from build123d import *

# Parameters (mm, degrees)
SKETCH1_R                = 4.05
BOSS_EXTRUDE1_DEPTH      = 8.1
BOSS_EXTRUDE2_DEPTH      = 1
FILLET1_R                = 10
SKETCH3_R                = 2
BOSS_EXTRUDE3_DEPTH      = 1.2
SKETCH4_R                = 0.4
BOSS_EXTRUDE4_DEPTH      = 3
BOSS_EXTRUDE5_START      = -0.5
SKETCH5_R                = 1.15
BOSS_EXTRUDE5_DEPTH      = 1.4
BOSS_EXTRUDE6_REACH      = 19.008
BOSS_EXTRUDE6_END_RADIUS = 4.05
SKETCH6_W                = 6
SKETCH6_H                = 4


with BuildPart() as part:
    # Sketch1 → Boss-Extrude1 (new body)
    with BuildSketch(Plane(origin=(0, 0, 0), x_dir=(1, 0, 0), z_dir=(0, 1, 0))):
        with Locations(Location((0, 0, 0), (0, 0, 270))):
            Circle(SKETCH1_R)
    extrude(amount=BOSS_EXTRUDE1_DEPTH)

    # Sketch2 → Boss-Extrude2 (add)
    with BuildSketch(Plane(origin=(0, 8.1, 0), x_dir=(1, 0, 0), z_dir=(0, 1, 0))):
        with BuildLine():
            ThreePointArc((-3.833548742, 1.30629401), (-2.205788092, -3.3966158), (2.752603705, -2.9708034))
            ThreePointArc((2.752603705, -2.9708034), (4.235286368, -2.750427127), (3.833548742, -1.30629401))
            ThreePointArc((3.833548742, -1.30629401), (2.205788092, 3.3966158), (-2.752603705, 2.9708034))
            ThreePointArc((-2.752603705, 2.9708034), (-4.235286368, 2.750427127), (-3.833548742, 1.30629401))
        make_face()
    extrude(amount=BOSS_EXTRUDE2_DEPTH)

    # Fillet1
    # the kernel refuses this fillet: 10 mm, written as the material it adds along each edge
    with BuildSketch(Plane(origin=(-2.752603705, 8.1, -2.9708034), x_dir=(0.8459561601363162, 0, -0.5332524497153475), z_dir=(0, 1, 0)), Plane(origin=(2.752603705, 8.1, 2.9708034), x_dir=(-0.8459561601363164, 0, 0.5332524497153472), z_dir=(0, 1, 0))) as fillet1_piece_1:
        with BuildLine():
            CenterArc((3.326797297, 9.829634829), FILLET1_R, 247.104601823, 12.304164649)
            ThreePointArc((-0.563702324, 0.617468271), (-0.214223286, 0.370473326), (0, 0))
            ThreePointArc((0, 0), (0.74439387, 0.068997894), (1.488787741, 0))
        make_face()
    extrude(amount=1)
    with BuildSketch(Plane(origin=(-3.833548742, 8.1, -1.30629401), x_dir=(-0.14306898445110627, 0, 0.9897127187664757), z_dir=(0, 1, 0)), Plane(origin=(3.833548742, 8.1, 1.30629401), x_dir=(0.14306898445110644, 0, -0.9897127187664757), z_dir=(0, 1, 0))) as fillet1_piece_2:
        with BuildLine():
            CenterArc((3.326797297, -9.829634829), FILLET1_R, 100.591233529, 12.304164649)
            ThreePointArc((-0.563702324, -0.617468271), (-0.214223286, -0.370473326), (0, 0))
            ThreePointArc((0, 0), (0.74439387, -0.068997894), (1.488787741, 0))
        make_face()
    extrude(amount=1)

    # Sketch3 → Boss-Extrude3 (add)
    with BuildSketch(Plane(origin=(0, 9.1, 0), x_dir=(1, 0, 0), z_dir=(0, 1, 0))):
        with Locations(Location((0, 0, 0), (0, 0, 270))):
            Circle(SKETCH3_R)
    extrude(amount=BOSS_EXTRUDE3_DEPTH)

    # Sketch4 → Boss-Extrude4 (add)
    with BuildSketch(Plane(origin=(0, 10.3, 0), x_dir=(1, 0, 0), z_dir=(0, 1, 0))):
        with Locations(Location((0, 0, 0), (0, 0, 270))):
            Circle(SKETCH4_R)
    extrude(amount=BOSS_EXTRUDE4_DEPTH)

    # Sketch5 → Boss-Extrude5 (add)
    with BuildSketch(Plane(origin=(0, 13.3, 0), x_dir=(1, 0, 0), z_dir=(0, 1, 0)).offset(BOSS_EXTRUDE5_START)):
        with Locations(Location((0, 0, 0), (0, 0, 270))):
            Circle(SKETCH5_R)
    extrude(amount=-BOSS_EXTRUDE5_DEPTH)

    # Boss-Extrude6: up to this cylinder (the profile starts outside it)
    boss_extrude6_end = Plane(origin=(0, 3.8, 0), z_dir=(0, -1, 0)) * Cylinder(BOSS_EXTRUDE6_END_RADIUS, 47.116, mode=Mode.PRIVATE)
    # Sketch6 → Boss-Extrude6 (add, up to the surface)
    with BuildSketch(Plane(origin=(5.4, 0, 0), x_dir=(0, 0, -1), z_dir=(1, 0, 0)), mode=Mode.PRIVATE) as boss_extrude6_sk1:
        with Locations((0, 3.8)):
            Rectangle(SKETCH6_W, SKETCH6_H)
    boss_extrude6_tool1 = extrude(boss_extrude6_sk1.sketch, amount=-BOSS_EXTRUDE6_REACH, mode=Mode.PRIVATE) - boss_extrude6_end
    add(boss_extrude6_tool1.solids().sort_by_distance((5.4, 3.8, 0))[0])


solid = part.part
Can you work these out from the model? Positions are in its coordinate system, mm. A direction names the side the tool comes from. Round coordinates to 2 decimals unless told otherwise and drop trailing zeros. Loops run counter-clockwise (first coordinate to the right, second up) from the corner with the lowest first, then second, coordinate; pieces in that order, holes last. Notation, with made-up numbers: (39.5, 23) - (62.5, 23) arc R28 cw to (62.5, 43) - close; hole circle Ø5 at (26, -40). An arc over 180 degrees is marked (long way). Use CSV: the item, a comma, the result in double quotes. Start each with the question number.
1) For pin 1 Ø3 at (x, z) = (4, -1) entering from +Y; pin 2 Ø5 at (x, y) = (3.5, 5) entering from +Z; pin 3 Ø1.5 at (y, z) = (9.5, -0.5) entering from -X, each with a flat end and sliding along its axis, tell me the tip position at first contact or that it passes through.
2) If we section it at A-A on z = 1.5: Write out the boundary of the cut face in (x, y).
3) If we section it at D-D on y = 11.25: Write out the boundary of the cut face in (x, z).
4) Please list where these lines run through material, in increasing order: probe 1 along Y at (x, z) = (1.25, 2.25); probe 2 along Z at (x, y) = (5.25, 2.75); probe 3 along X at (y, z) = (2.75, 1.5). Write a range as [from, to].
5) If we section it at C-C on x = 2.25: Write out the boundary of the cut face in (y, z).
6) For faces 5 (the cylindrical face through (0.345, 12.11, 1.097)), 6 (the cylindrical face through (4.146, 8.593, 0.886)), 7 (the flat face through (-0.5, 11.4, 0.24)), which set-ups out of +Z, -Z, +X, -X, +Y, -Y let a thin tool reach every point of the face, with its end or its side?
7) We'd pull the mould along Y, two halves only. Please class faces 1 (the flat face through (-0.4, 10.3, 0.4)), 2 (the flat face through (-1, 9.1, 2)), 3 (the flat face through (4, 8.1, 2)), 4 (the flat face through (4, 4, -3)): released by +Y, released by -Y, zero draft, split by the parting line, or undercut.
8) If we section it at B-B on x = -1: Write out the boundary of the cut face in (y, z), plus the area to 3 significant figures.
Geometry results:
1,pin 1,"stops at y = 9.1"
1,pin 2,"stops at z = 3.92"
1,pin 3,"stops at x = -4.19"
2,outline,"(-3.76, 0) - (3.76, 0) - (3.76, 1.8) - (5.4, 1.8) - (5.4, 5.8) - (3.76, 5.8) - (3.76, 8.1) - (4.26, 8.1) - (4.26, 9.1) - (1.32, 9.1) - (1.32, 10.3) - (-1.32, 10.3) - (-1.32, 9.1) - (-3.76, 9.1) - close"
3,outline,"circle Ø0.8 at (0, 0)"
4,probe 1,"y = [0, 9.1]"
4,probe 2,"z = [-3, 3]"
4,probe 3,"x = [-3.76, 5.4]"
5,outline,"(0, -3.37) - (9.1, -3.37) - (9.1, 3.5) - (8.1, 3.5) - (8.1, 3.37) - (0, 3.37) - close"
6,face 5,"+Y"
6,face 6,"-Z, +X, +Y"
6,face 7,"none"
7,face 1,"undercut"
7,face 2,"released by +Y"
7,face 3,"undercut"
7,face 4,"zero draft"
8,outline,"(0, -3.92) - (9.1, -3.92) - (9.1, -1.73) - (10.3, -1.73) - (10.3, 1.73) - (9.1, 1.73) - (9.1, 3.92) - (0, 3.92) - close; (11.4, -0.57) - (12.8, -0.57) - (12.8, 0.57) - (11.4, 0.57) - close"
8,area,"77.2 mm2"
